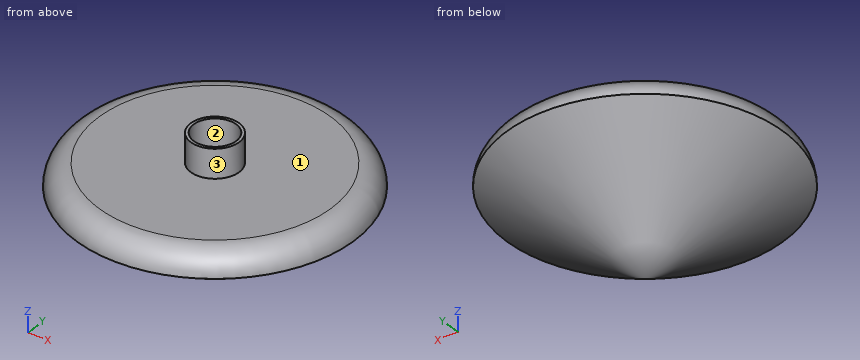
```python
from build123d import *

# Parameters (mm, degrees)
F2_R     = 4.7625
F3_DEPTH = 9.525
F4_R     = 5.07999


# Not quite as in the source:
# - a fillet or chamfer is up to 0.001 mm smaller than in the source, because OpenCascade refuses the exact size


with BuildPart() as f1:
    # F0 (on Front) → F1 (revolve)
    with BuildSketch(Plane.XZ):
        Polygon((0, 31.392690606), (0, 0), (31.0912281275, 19.8785602432), (31.0912281275, 24.9585602432), (5.4195728153, 24.9585602432), (5.4195728153, 31.392690606), align=None)
    revolve(axis=Axis((0, 0, 15.696345303), (0, 0, -1)))

    # F2 (on face) → F3 (cut)
    with BuildSketch(Plane.XY.offset(31.392690606)):
        Circle(F2_R)
    extrude(amount=-F3_DEPTH, mode=Mode.SUBTRACT)

    # F4 (radius 5.08 in the source; OpenCascade refuses exactly that, so slightly less here)
    f4_edges = [f1.edges().sort_by_distance(p)[0] for p in [
        (-31.091228, 0, 24.95856),
    ]]
    fillet(f4_edges, radius=F4_R)


solid = f1.part
```
The listing builds one solid part. Answer for the finished solid, in the listing's coordinates (mm). Face numbers are marked on the shaded views. Round coordinates to 2 decimals unless told otherwise and drop trailing zeros. Order: outer loops, then holes, each group sorted by start corner. A loop starts at its lowest first (then second) coordinate and runs counter-clockwise, first axis right, second up. Notation, with made-up numbers: (8.5, -6) -> (63.5, -6) arc R14 cw to (63.5, 14) -> close; hole circle Ø4 at (55.25, 52.25). An arc over 180 degrees is marked (long way). Answer as CSV lines item,"result". Start each with the question number.
(1) The part is cut by section C-C (z = 21). Determine the outline of the cut face in (x, y), then the cut area to 3 significant figures.
(2) For a pull along X with two mould halves and no side action, classify the marked faces 1, 2 and 3 as +X half, -X half, draft (parallel to the pull), parting line (faces both ways), or undercut.
(3) The part is cut by section B-B (z = 8). Determine the outline of the cut face in (x, y), then the cut area to 3 significant figures.
(4) The part is cut by section A-A (z = 29.5). Determine the outline of the cut face in (x, y) (1 decimal).
(5) Find the intervals of material crossed by probe 1 along Y at (x, z) = (0, 29); probe 2 along Y at (x, z) = (18, 17.5); probe 3 along Z at (x, y) = (12, -2.5), in increasing order. Write a range as from..to.
(6) Flat-ended cylindrical pins translate along their axes: pin 1 Ø2 at (x, y) = (11.5, 13) entering from -Z; pin 2 Ø3 at (x, z) = (-7.5, 12.5) entering from -Y; pin 3 Ø8.5 at (x, y) = (0, 0) entering from +Z. Find the tip coordinate at first contact, or state that the pin passes through.
Evaluation:
1,outline,"circle Ø61.93 at (0, 0)"
1,area,"3,010 mm²"
2,face 1,"draft"
2,face 2,"undercut"
2,face 3,"parting line"
3,outline,"circle Ø25.02 at (0, 0)"
3,area,"492 mm²"
4,outline,"circle Ø10.8 at (0, 0); hole circle Ø9.5 at (0, 0)"
5,probe 1,"-5.42..-4.76, 4.76..5.42"
5,probe 2,"-20.62..20.62"
5,probe 3,"7.84..24.96"
6,pin 1,"z = 10.46"
6,pin 2,"y = -20.63"
6,pin 3,"z = 21.87"
